from build123d import *

# Parameters (mm, degrees)
SKETCH3_R           = 11.1125
BOSS_EXTRUDE1_DEPTH = 6.35
SKETCH5_W           = 31.75
SKETCH5_H           = 6.35
BOSS_EXTRUDE2_DEPTH = 38.1
FILLET1_R           = 4.7625
SKETCH6_R           = 1.777000002
CUT_EXTRUDE1_DEPTH  = 7.35


with BuildPart() as part:
    # Sketch3 → Boss-Extrude1 (new body)
    with BuildSketch(Plane(origin=(0, 0, 0), x_dir=(0, 0, -1), z_dir=(1, 0, 0))):
        with BuildLine():
            Line((0, 0), (31.75, 0))
            Line((31.75, 0), (31.75, 49.2125))
            ThreePointArc((31.75, 49.2125), (15.875, 65.0875), (0, 49.2125))
            Line((0, 49.2125), (0, 0))
        make_face()
        with Locations((15.875, 49.2125)):
            Circle(SKETCH3_R, mode=Mode.SUBTRACT)
    extrude(amount=BOSS_EXTRUDE1_DEPTH)

    # Sketch5 → Boss-Extrude2 (add)
    with BuildSketch(Plane(origin=(6.35, 0, 0), x_dir=(0, 0, -1), z_dir=(1, 0, 0))):
        with Locations((15.875, -3.175)):
            Rectangle(SKETCH5_W, SKETCH5_H)
    extrude(amount=-BOSS_EXTRUDE2_DEPTH)

    # Fillet1
    fillet1_edges = [part.edges().sort_by_distance(p)[0] for p in [
        (0, 0, -15.875),
    ]]
    fillet(fillet1_edges, radius=FILLET1_R)

    # Sketch6 → Cut-Extrude1 (cut, through all)
    with BuildSketch(Plane(origin=(0, 0, 0), x_dir=(1, 0, 0), z_dir=(0, 1, 0))):
        with Locations((-11.1125, 6.35)):
            Circle(SKETCH6_R)
        with Locations((-25.4, 15.875)):
            Circle(SKETCH6_R)
        with Locations((-11.1125, 25.4)):
            Circle(SKETCH6_R)
    extrude(amount=-CUT_EXTRUDE1_DEPTH, mode=Mode.SUBTRACT)


solid = part.part
Geometry: final body of the model. Coordinates: model frame, mm. A direction names the side the tool comes from. Give positions to 0.01 mm unless a question says otherwise; leave off trailing zeros. Write each loop counter-clockwise with the first axis right and the second up, starting at its lowest first coordinate (ties: lowest second). Pieces come first, ordered by that corner, then holes. Notation, with made-up numbers: (44, 18) - (62, 18) arc R32 cw to (62, 50) - close; hole circle Ø3 at (43.25, 73.25). An arc over 180 degrees is marked (long way). Return JSON: item names as keys, results as strings. Group by question number.
1) Set-up query: faces 1 (the flat face through (-31.75, -3, -16)), 2 (the flat face through (0, 29, -16)). Return all of +Z, -Z, +X, -X, +Y, -Y with unobstructed straight access to the full face (end or side cutting, diameter ignored); none if empty.
2) Section B-B on z = -25.4. State how many separate pieces and enclosed holes the cut face has, plus the area to 3 significant figures.
3) Mould query, pull axis Z, two halves, no side actions, for faces 3 (the flat face through (2, 11, -31.75)), 4 (the flat face through (-12, -6.35, -16)), 5 (the cylindrical face through (-9.418, -3.131, -6.884)), 6 (the flat face through (2, 11, 0)). Classes: released by +Z, released by -Z, zero draft, split by the parting line, or undercut.
4) First-contact query: P1, Ø3, axis at x = -11.11, z = -6.35, coming from the +Y side; P2, Ø12, axis at x = 0, z = -28, coming from the +Y side. Flat tips, straight axial feed; report the tip coordinate or a pass-through.
5) Section A-A on x = -24.5. Return the cut outline in (y, z), plus the area to 3 significant figures.
6) Line query: line 1 (X direction, y = 37, z = -17.5); line 2 (Y direction, x = -12, z = -19); line 3 (Y direction, x = 5.5, z = -19). Output: solid intervals per line, ascending.
7) Section C-C on x = -18. Return the cut outline in (y, z).
Filled in:
{
 "1": {"face 1": "+Z, -Z, -X, +Y, -Y", "face 2": "+Z, -Z, -X, +Y"},
 "2": {"separate pieces": "3", "enclosed holes": "0", "area": "545 mm^2"},
 "3": {"face 3": "released by -Z", "face 4": "zero draft", "face 5": "undercut", "face 6": "released by +Z"},
 "4": {"P1": "passes through", "P2": "stops at y = 63.86"},
 "5": {"outline": "(-6.35, -31.75) - (0, -31.75) - (0, -17.41) - (-6.35, -17.41) - close; (-6.35, -14.34) - (0, -14.34) - (0, 0) - (-6.35, 0) - close", "area": "182 mm^2"},
 "6": {"line 1": "x = 0 to 6.35", "line 2": "y = -6.35 to 0", "line 3": "y = -6.35 to 38.55, 59.88 to 64.78"},
 "7": {"outline": "(-6.35, -31.75) - (0, -31.75) - (0, 0) - (-6.35, 0) - close"}
}
